Read the model definition and answer for the solid it produces. Units are mm, in the model's axes. Face numbers are marked on the shaded views. Round coordinates to 2 decimals unless told otherwise and drop trailing zeros. Order: outer loops, then holes, each group sorted by start corner. A loop starts at its lowest first (then second) coordinate and runs counter-clockwise, first axis right, second up. Notation, with made-up numbers: (21, 54.25) -> (50, 54.25) arc R4 ccw to (50, 59.25) -> close; hole circle Ø6 at (70, 83). An arc over 180 degrees is marked (long way). Answer as a JSON object with one key per item and string values. Group by question number.
Item 1: Section A-A, the plane y = -48.5 is taken. Write down the section's boundary in (x, z), plus the area to 3 significant figures.
Item 2: Given P1, Ø1, axis at x = 3, y = 51.5, coming from the +Z side; P2, Ø1, axis at x = -2.5, z = -14.5, coming from the -Y side; P3, Ø3, axis at x = 2, y = -46.5, coming from the -Z side, each flat-ended and moving along its own axis, determine where each tip first touches the part or whether it passes through.
Item 3: Consider probe 1 along Z at (x, y) = (1.5, 45.5); probe 2 along Z at (x, y) = (3, 46); probe 3 along Y at (x, z) = (0, -24) (3 decimals). Determine where each line is inside the solid, lowest interval first. Write a range as from..to.
Item 4: The mould has two halves that part along Z. Classify the marked faces 1, 2 and 3: pulls with the +Z half, pulls with the -Z half, needs draft (parallel to the pull), parting line crosses it, or undercut.
Item 5: Section B-B, the plane z = -17.5 is taken. Write down the section's boundary in (x, y), plus the area to 3 significant figures.
from build123d import *

# Parameters (mm, degrees)
BOSS_EXTRUDE1_DEPTH      = 57.15
BOSS_EXTRUDE1_2_DEPTH    = 57.15
BOSS_EXTRUDE2_DEPTH      = 50.8
BOSS_EXTRUDE3_DEPTH      = 0.6
BOSS_EXTRUDE3_DEPTH_BACK = 3.521
SKETCH3_R                = 3.175
SKETCH4_W                = 1.016
SKETCH4_H                = 10.16
CUT_EXTRUDE1_DEPTH       = 74.455759645
SKETCH5_W                = 7.62
SKETCH5_H                = 2
CUT_EXTRUDE2_DEPTH       = 85.988054602
BOSS_EXTRUDE6_DEPTH      = 0.6
BOSS_EXTRUDE6_DEPTH_BACK = 3.521
SKETCH6_R                = 3.175
BOSS_EXTRUDE7_START      = 3.302
SKETCH7_R                = 1.7145
BOSS_EXTRUDE7_DEPTH      = 2.54
SKETCH8_W                = 2.54
SKETCH8_H                = 7.76
BOSS_EXTRUDE8_DEPTH      = 7.62


with BuildPart() as part:
    # Sketch1 → Boss-Extrude1 (new, symmetric)
    with BuildSketch(Plane(origin=(0, 0, 0), x_dir=(1, 0, 0), z_dir=(0, 1, 0))):
        with BuildLine():
            Line((-3.81, 25.4), (-3.81, 22.479))
            Line((-3.81, 22.479), (-2.794, 22.479))
            ThreePointArc((-2.794, 22.479), (-2.630731947, 22.538424711), (-2.543858831, 22.688893363))
            Line((-2.543858831, 22.688893363), (-2.352506152, 23.774108332))
            ThreePointArc((-2.352506152, 23.774108332), (-2.178759919, 24.075045635), (-1.852223813, 24.193895058))
            Line((-1.852223813, 24.193895058), (1.852223813, 24.193895058))
            ThreePointArc((1.852223813, 24.193895058), (2.178759919, 24.075045635), (2.352506152, 23.774108332))
            Line((2.352506152, 23.774108332), (2.543858831, 22.688893363))
            ThreePointArc((2.543858831, 22.688893363), (2.630731947, 22.538424711), (2.794, 22.479))
            Line((2.794, 22.479), (3.81, 22.479))
            Line((3.81, 22.479), (3.81, 25.4))
            Line((3.81, 25.4), (-3.81, 25.4))
        make_face()
    extrude(amount=BOSS_EXTRUDE1_DEPTH, both=True)



with BuildPart() as body_2:
    # Sketch1 → Boss-Extrude1 2 (new, symmetric)
    with BuildSketch(Plane(origin=(0, 0, 0), x_dir=(1, 0, 0), z_dir=(0, 1, 0))):
        with BuildLine():
            Line((-2.278486426, -24.193895058), (-2.543858831, -22.688893363))
            ThreePointArc((-2.543858831, -22.688893363), (-2.630731947, -22.538424711), (-2.794, -22.479))
            Line((-2.794, -22.479), (-3.81, -22.479))
            Line((-3.81, -22.479), (-3.81, -25.4))
            Line((-3.81, -25.4), (3.81, -25.4))
            Line((3.81, -25.4), (3.81, -22.479))
            Line((3.81, -22.479), (2.794, -22.479))
            ThreePointArc((2.794, -22.479), (2.630731947, -22.538424711), (2.543858831, -22.688893363))
            Line((2.543858831, -22.688893363), (2.278486426, -24.193895058))
            ThreePointArc((2.278486426, -24.193895058), (2.070186355, -24.241918271), (1.860572408, -24.2))
            Line((1.860572408, -24.2), (-2.146199428, -24.2))
            ThreePointArc((-2.146199428, -24.2), (-2.212542712, -24.201276643), (-2.278486426, -24.193895058))
        make_face()
    extrude(amount=BOSS_EXTRUDE1_2_DEPTH, both=True)


with BuildPart() as part_1:
    add(part.part)

    add(body_2.part)  # Boss-Extrude2 merges body 2
    # Sketch2 → Boss-Extrude2 (add)
    with BuildSketch(Plane.XY.offset(25.4)):
        Polygon((-3.81, 57.15), (3.81, 57.15), (3.81, 55.95), (0.6, 55.412830225), (0.6, 48.727169775), (3.81, 48.19), (3.81, 46.99), (-3.81, 46.99), (-3.81, 48.19), (-0.6, 48.727169775), (-0.6, 55.412830225), (-3.81, 55.95), align=None)
    extrude(amount=-BOSS_EXTRUDE2_DEPTH)

    # Sketch3 → Boss-Extrude3 (add, two sides: drawn at the far end of the back side and taken through both)
    with BuildSketch(Plane.XY.offset(25.4).offset(-BOSS_EXTRUDE3_DEPTH_BACK)):
        with BuildLine():
            Line((-5.08, -54.61), (5.08, -54.61))
            Line((5.08, -54.61), (5.08, -62.865))
            ThreePointArc((5.08, -62.865), (0, -67.945), (-5.08, -62.865))
            Line((-5.08, -62.865), (-5.08, -54.61))
        make_face()
        with Locations((0, -62.865)):
            Circle(SKETCH3_R, mode=Mode.SUBTRACT)
    extrude(amount=BOSS_EXTRUDE3_DEPTH + BOSS_EXTRUDE3_DEPTH_BACK)

    # Sketch4 → Cut-Extrude1 (cut, through all)
    with BuildSketch(Plane.ZY.offset(5.08)):
        with Locations((22.387, -62.865)):
            Rectangle(SKETCH4_W, SKETCH4_H)
    cut_extrude1 = extrude(amount=-CUT_EXTRUDE1_DEPTH, mode=Mode.SUBTRACT)

    # Sketch5 → Cut-Extrude2 (cut, through all)
    with BuildSketch(Plane.XY.offset(25.4)):
        with Locations((0, -55.61)):
            Rectangle(SKETCH5_W, SKETCH5_H)
    cut_extrude2 = extrude(amount=CUT_EXTRUDE2_DEPTH, mode=Mode.SUBTRACT)

    # Sketch6 → Boss-Extrude6 (add, two sides: drawn at the far end of the back side and taken through both)
    with BuildSketch(Plane(origin=(0, 0, -25.4), x_dir=(-1, 0, 0), z_dir=(0, 0, -1)).offset(-BOSS_EXTRUDE6_DEPTH_BACK)):
        with BuildLine():
            Line((-5.08, -54.61), (5.08, -54.61))
            Line((5.08, -54.61), (5.08, -62.865))
            ThreePointArc((5.08, -62.865), (0, -67.945), (-5.08, -62.865))
            Line((-5.08, -62.865), (-5.08, -54.61))
        make_face()
        with Locations(Location((0, -62.865, 0), (0, 0, 180))):
            Circle(SKETCH6_R, mode=Mode.SUBTRACT)
    extrude(amount=BOSS_EXTRUDE6_DEPTH + BOSS_EXTRUDE6_DEPTH_BACK)

    # Mirror5: Cut-Extrude1 across plane
    add(cut_extrude1.mirror(Plane.XY), mode=Mode.SUBTRACT)

    # Mirror6: Cut-Extrude2 across plane
    add(cut_extrude2.mirror(Plane.XY), mode=Mode.SUBTRACT)

    # Sketch7 → Boss-Extrude7 (add)
    with BuildSketch(Plane.XY.offset(BOSS_EXTRUDE7_START)):
        with BuildLine():
            Line((3.81, 43.18), (3.81, 46.99))
            Line((3.81, 46.99), (-3.81, 46.99))
            Line((-3.81, 46.99), (-3.81, 43.18))
            ThreePointArc((-3.81, 43.18), (0, 39.37), (3.81, 43.18))
        make_face()
        with Locations((0, 43.18)):
            Circle(SKETCH7_R, mode=Mode.SUBTRACT)
    boss_extrude7 = extrude(amount=BOSS_EXTRUDE7_DEPTH)

    # Mirror7: Boss-Extrude7 across plane
    add(boss_extrude7.mirror(Plane.XY))

    # Sketch8 → Boss-Extrude8 (add)
    with BuildSketch(Plane.ZY.offset(3.81)):
        with Locations((4.572, 52.07)):
            Rectangle(SKETCH8_W, SKETCH8_H)
    boss_extrude8 = extrude(amount=-BOSS_EXTRUDE8_DEPTH)

    # Mirror8: Boss-Extrude8 across plane
    add(boss_extrude8.mirror(Plane.XY))


solid = part_1.part
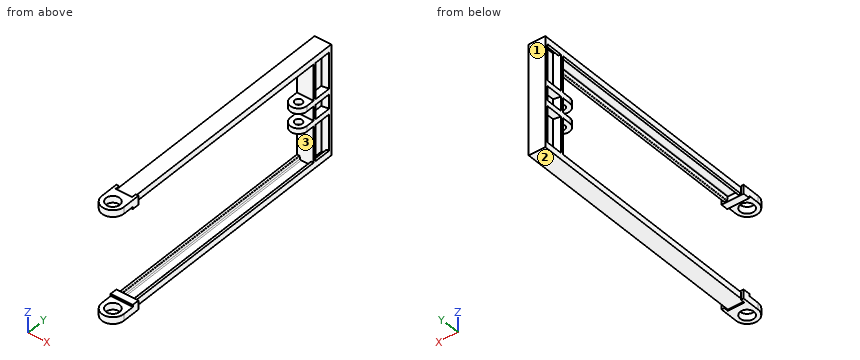
Values found:
{
 "1": {"outline": "(-3.81, -25.4) -> (3.81, -25.4) -> (3.81, -22.48) -> (2.79, -22.48) arc R0.25 ccw to (2.54, -22.69) -> (2.35, -23.77) arc R0.51 cw to (1.85, -24.19) -> (-1.85, -24.19) arc R0.51 cw to (-2.35, -23.77) -> (-2.54, -22.69) arc R0.25 ccw to (-2.79, -22.48) -> (-3.81, -22.48) -> close; (-3.81, 22.48) -> (-2.79, 22.48) arc R0.25 ccw to (-2.54, 22.69) -> (-2.28, 24.19) arc R0.51 cw to (-2.15, 24.2) -> (1.86, 24.2) arc R0.51 cw to (2.28, 24.19) -> (2.54, 22.69) arc R0.25 ccw to (2.79, 22.48) -> (3.81, 22.48) -> (3.81, 25.4) -> (-3.81, 25.4) -> close", "area": "27.8 mm2"},
 "2": {"P1": "z = 25.4", "P2": "y = 46.99", "P3": "z = -25.4"},
 "3": {"probe 1": "-25.4..-24.19, -5.84..-3.3, 3.3..5.84, 24.2..25.4", "probe 2": "-25.4..-22.48, -5.84..-3.3, 3.3..5.84, 22.48..25.4", "probe 3": "-67.945..-66.04, -59.69..-54.61, 46.99..57.15"},
 "4": {"face 1": "needs draft", "face 2": "pulls with the -Z half", "face 3": "undercut"},
 "5": {"outline": "(-3.81, 46.99) -> (3.81, 46.99) -> (3.81, 48.19) -> (0.6, 48.73) -> (0.6, 55.41) -> (3.81, 55.95) -> (3.81, 57.15) -> (-3.81, 57.15) -> (-3.81, 55.95) -> (-0.6, 55.41) -> (-0.6, 48.73) -> (-3.81, 48.19) -> close", "area": "31.0 mm2"}
}
